from build123d import *

# Parameters (mm, degrees)
ESQUISSE1_R                  = 5.9
BOSS_EXTRU_1_DEPTH           = 5
COQUE1_T                     = -0.5
ESQUISSE2_R                  = 5.9
ESQUISSE2_R_2                = 1.25
BOSS_EXTRU_2_DEPTH           = 1.5
ESQUISSE3_R                  = 4.5
BOSS_EXTRU_3_DEPTH           = 4
ESQUISSE4_R                  = 0.45
BOSS_EXTRU_4_DEPTH           = 2.6
ESQUISSE5_R                  = 0.65
BOSS_EXTRU_5_DEPTH           = 0.9
BOSS_EXTRU_5_DRAFT           = -12
BOSS_EXTRU_5_PROFILE_2_DEPTH = 0.9
BOSS_EXTRU_5_PROFILE_2_DRAFT = -12


with BuildPart() as part:
    # Esquisse1 → Boss.-Extru.1 (new body)
    with BuildSketch(Plane(origin=(0, 0, 0), x_dir=(1, 0, 0), z_dir=(0, 1, 0))):
        with Locations(Location((0, 0, 0), (0, 0, 270))):
            Circle(ESQUISSE1_R)
    extrude(amount=BOSS_EXTRU_1_DEPTH)

    # Coque1
    coque1_openings = [part.faces().sort_by_distance(p)[0] for p in [
        (0, 5, 0),
    ]]
    offset(amount=COQUE1_T, openings=coque1_openings, kind=Kind.INTERSECTION)

    # Esquisse2 → Boss.-Extru.2 (add)
    with BuildSketch(Plane(origin=(0, 5, 0), x_dir=(1, 0, 0), z_dir=(0, 1, 0))):
        with Locations(Location((0, 0, 0), (0, 0, 270))):
            Circle(ESQUISSE2_R)
        with Locations(Location((0, 0, 0), (0, 0, 270))):
            Circle(ESQUISSE2_R_2, mode=Mode.SUBTRACT)
    extrude(amount=BOSS_EXTRU_2_DEPTH)

    # Esquisse3 → Boss.-Extru.3 (add)
    with BuildSketch(Plane(origin=(0, 0.5, 0), x_dir=(1, 0, 0), z_dir=(0, 1, 0))):
        with Locations(Location((0, 0, 0), (0, 0, 270))):
            Circle(ESQUISSE3_R)
    extrude(amount=BOSS_EXTRU_3_DEPTH)

    # Esquisse4 → Boss.-Extru.4 (add)
    with BuildSketch(Plane.XZ):
        with Locations(Location((0, 3.65, 0), (0, 0, 90))):
            Circle(ESQUISSE4_R)
        with Locations(Location((0, -3.647, 0), (0, 0, 90))):
            Circle(ESQUISSE4_R)
    extrude(amount=BOSS_EXTRU_4_DEPTH)


with BuildPart() as boss_extru_5_tool:
    # Esquisse5 → Boss.-Extru.5 (with draft: the straight prism first)
    with BuildSketch(Plane(origin=(0, -1.7, 0), x_dir=(1, 0, 0), z_dir=(0, 1, 0))):
        with Locations((0, -3.65)):
            Circle(ESQUISSE5_R)
    extrude(amount=-BOSS_EXTRU_5_DEPTH)
    # Boss.-Extru.5: the draft: its side faces are tilted about the plane it starts from
    boss_extru_5_sides = [boss_extru_5_tool.faces().sort_by_distance(p)[0] for p in [
        (-0.65, -2.15, 3.65),
    ]]
    draft(boss_extru_5_sides, Plane(origin=(0, -1.7, 0), x_dir=(1, 0, 0), z_dir=(0, 1, 0)), BOSS_EXTRU_5_DRAFT)


with BuildPart() as part_1:
    add(part.part)

    # Boss.-Extru.5: add boss_extru_5_tool
    add(boss_extru_5_tool.part)


with BuildPart() as boss_extru_5_profile_2_tool:
    # Esquisse5 → Boss.-Extru.5 profile 2 (with draft: the straight prism first)
    with BuildSketch(Plane(origin=(0, -1.7, 0), x_dir=(1, 0, 0), z_dir=(0, 1, 0))):
        with Locations((0, 3.647)):
            Circle(ESQUISSE5_R)
    extrude(amount=-BOSS_EXTRU_5_PROFILE_2_DEPTH)
    # Boss.-Extru.5 profile 2: the draft: its side faces are tilted about the plane it starts from
    boss_extru_5_profile_2_sides = [boss_extru_5_profile_2_tool.faces().sort_by_distance(p)[0] for p in [
        (-0.65, -2.15, -3.647),
    ]]
    draft(boss_extru_5_profile_2_sides, Plane(origin=(0, -1.7, 0), x_dir=(1, 0, 0), z_dir=(0, 1, 0)), BOSS_EXTRU_5_PROFILE_2_DRAFT)


with BuildPart() as part_2:
    add(part_1.part)

    # Boss.-Extru.5 profile 2: add boss_extru_5_profile_2_tool
    add(boss_extru_5_profile_2_tool.part)


solid = part_2.part
Here's how the part is built. I have some questions about the finished solid (model axes, mm). A direction names the side the tool comes from. Round coordinates to 2 decimals unless told otherwise and drop trailing zeros. Write each loop counter-clockwise with the first axis right and the second up, starting at its lowest first coordinate (ties: lowest second). Pieces come first, ordered by that corner, then holes.
1. Suppose I cut it at C-C (x = -3.5). List the corners of the cut face in (y, z) for me, and give its area (3 significant figures).
2. I need wall thicknesses on L1, parallel to X at y = 2.05, z = 0; L2, parallel to Y at x = 2, z = 0.75; L3, parallel to X at y = 5.7, z = 0. Which ranges of each line are inside material? Lowest first, please.
3. For faces 4 (the cylindrical face through (-1.22, 5.74, -0.27)), 5 (the flat face through (0, -2.6, 3.6)), 6 (the flat face through (0, 4.5, 0)), which set-ups out of +Z, -Z, +X, -X, +Y, -Y let a thin tool reach every point of the face, with its end or its side?
4. Suppose I cut it at B-B (z = 0). List the corners of the cut face in (x, y) for me, and give its area (4 significant figures).
5. Suppose I cut it at A-A (y = 3). List the corners of the cut face in (x, z) for me, and give its area (3 significant figures).
6. Will these pins go through, and if not, where does the flat tip stop? pin 1 Ø2 at (x, z) = (0, 0) entering from -Y; pin 2 Ø1.5 at (x, y) = (-3, 0) entering from -Z.
7. If we mould it in two halves opening along Z, with no side actions, what happens to faces 1 (the flat face through (0, -2.6, -3.7)), 2 (the conical face through (-0.07, -2.24, 3.12)), 3 (the cylindrical face through (-5.76, 3.2, -1.28))? For each: released by +Z, released by -Z, zero draft, split by the parting line, or undercut.
Answer sheet:
1. outline: (0, -4.75) - (6.5, -4.75) - (6.5, 4.75) - (0, 4.75) - close; hole (0.5, -4.11) - (5, -4.11) - (5, 4.11) - (0.5, 4.11) - (0.5, 2.83) - (4.5, 2.83) - (4.5, -2.83) - (0.5, -2.83) - close
1. area: 47.4 mm2
2. L1: x = -5.9 to -5.4, -4.5 to 4.5, 5.4 to 5.9
2. L2: y = 0 to 4.5, 5 to 6.5
2. L3: x = -5.9 to -1.25, 1.25 to 5.9
3. face 4: +Y
3. face 5: +Z, -Z, +X, -X, -Y
3. face 6: none
4. outline: (-5.9, 0) - (5.9, 0) - (5.9, 6.5) - (1.25, 6.5) - (1.25, 5) - (5.4, 5) - (5.4, 0.5) - (4.5, 0.5) - (4.5, 4.5) - (-4.5, 4.5) - (-4.5, 0.5) - (-5.4, 0.5) - (-5.4, 5) - (-1.25, 5) - (-1.25, 6.5) - (-5.9, 6.5) - close
4. area: 60.35 mm2
5. outline: circle Ø11.8 at (0, 0); circle Ø9 at (0, 0); hole circle Ø10.8 at (0, 0)
5. area: 81.4 mm2
6. pin 1: stops at y = 0
6. pin 2: stops at z = -5.45
7. face 1: zero draft
7. face 2: undercut
7. face 3: split by the parting line
